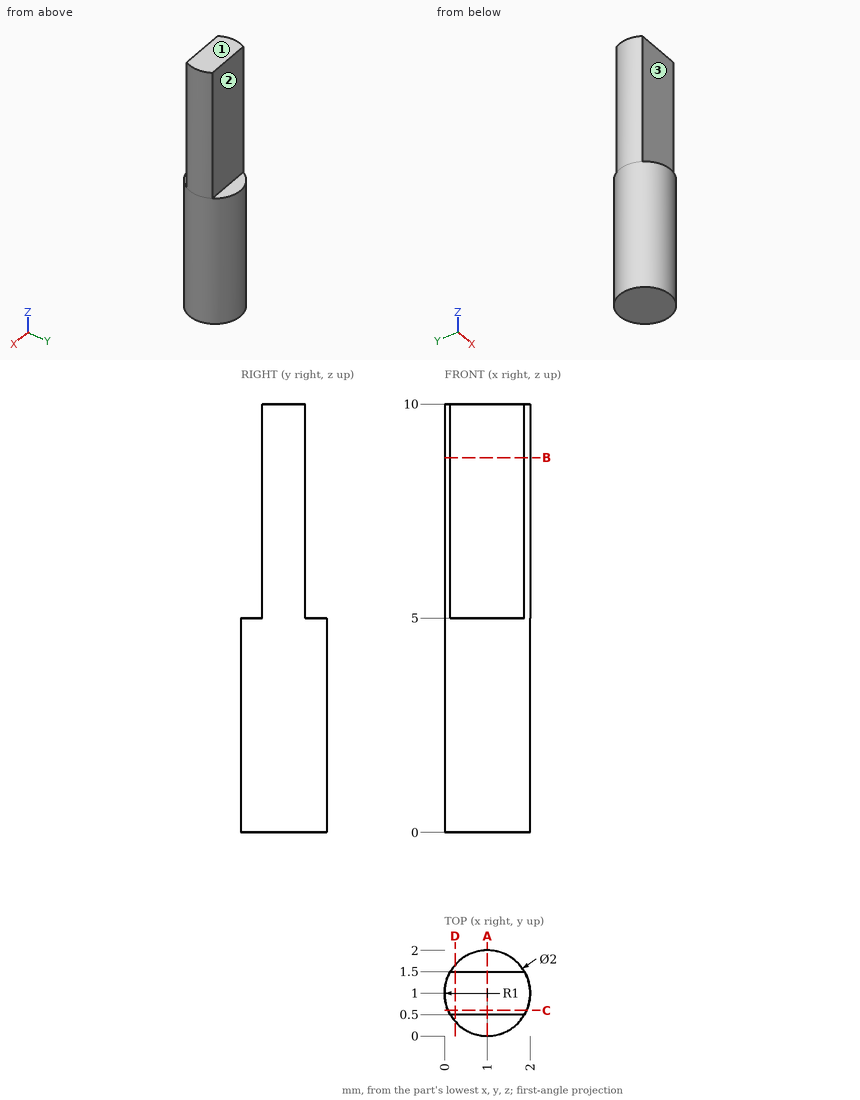
Input: dimensioned drawing with shaded views. Units: mm. Origin: part minimum x, y, z. A direction names the side the tool comes from. Round coordinates to 2 decimals unless told otherwise and drop trailing zeros. Loops run counter-clockwise (first coordinate to the right, second up) from the corner with the lowest first, then second, coordinate; pieces in that order, holes last. Notation, with made-up numbers: M 0.5,86.25 L 35.5,86.25 A9 cw 35.5,103.25 Z; hole C 54,-21.75 d7. An arc over 180 degrees is marked long. One line per question, with ' | ' between items.
(1) Cut plane D-D on x = 0.25. Return the cut outline in (y, z).
Check result:
outline: M 0.34,0 L 1.66,0 L 1.66,5 L 1.5,5 L 1.5,10 L 0.5,10 L 0.5,5 L 0.34,5 Z
(2) Contact query for flat-ended pins moving along their axis: P1, Ø0.5, axis at x = 0.5, z = 8.5, coming from the +Y side; P2, Ø0.6, axis at x = 0.5, y = 2, coming from the +Z side. Output: stop coordinate, or through.
Check result:
P1: stops at y = 1.5 | P2: stops at z = 5
(3) Cut plane C-C on y = 0.6. Return the cut outline in (x, z), plus the area to 3 significant figures.
Check result:
outline: M 0.08,0 L 1.92,0 L 1.92,10 L 0.08,10 Z | area: 18.3 mm2
(4) Cut plane B-B on z = 8.75. Return the cut outline in (x, y).
Check result:
outline: M 0.13,0.5 L 1.87,0.5 A1 ccw 1.87,1.5 L 0.13,1.5 A1 ccw Z
(5) Cut plane A-A on x = 1. Return the cut outline in (y, z).
Check result:
outline: M 0,0 L 2,0 L 2,5 L 1.5,5 L 1.5,10 L 0.5,10 L 0.5,5 L 0,5 Z
(6) Material intervals for line 1 along Z through (x, y) = (1.05, 0.35); line 2 along Y through (x, z) = (0.3, 6); line 3 along X through (y, z) = (0.95, 7.75), sorted ascending. Write a range as from..to.
Check result:
line 1: z = 0..5 | line 2: y = 0.5..1.5 | line 3: x = 0..2
(7) Access query for the marked faces 1, 2 and 3. Directions: +Z, -Z, +X, -X, +Y, -Y. A direction counts if a zero-diameter tool reaches every point of the face in a straight line with its end or side. Return the directions, or none.
Check result:
face 1: +Z, +X, -X, +Y, -Y | face 2: +Z, +X, -X, +Y | face 3: +Z, +X, -X, -Y
